Check sheet for the modelled part. Datum: model origin and axes. Units: mm. Face numbers are marked on the shaded views. A direction names the side the tool comes from. Give positions to 0.01 mm unless a question says otherwise; leave off trailing zeros. Order: outer loops, then holes, each group sorted by start corner. A loop starts at its lowest first (then second) coordinate and runs counter-clockwise, first axis right, second up. Notation, with made-up numbers: (-15, 52.5) - (-3, 52.5) arc R21 cw to (-3, 76.5) - close; hole circle Ø4 at (14, -23.75). An arc over 180 degrees is marked (long way). Answer in a Markdown table with one row per item.
from build123d import *

# Parameters (mm, degrees)
SKETCH1_W           = 120
SKETCH1_H           = 86
SKETCH1_W_2         = 10
SKETCH1_H_2         = 60
BOSS_EXTRUDE1_DEPTH = 470


with BuildPart() as part:
    # Sketch1 → Boss-Extrude1 (new body)
    with BuildSketch(Plane(origin=(0, 0, 0), x_dir=(1, 0, 0), z_dir=(0, 1, 0))):
        with BuildLine():
            Line((60, 74.46), (-69.377570777, 74.46))
            ThreePointArc((-69.377570777, 74.46), (-97.633626185, 65.17182404), (-117.46, 43))
            Line((-117.46, 43), (-117.46, -43))
            ThreePointArc((-117.46, -43), (-97.633626185, -65.17182404), (-69.377570777, -74.46))
            Line((-69.377570777, -74.46), (60, -74.46))
            ThreePointArc((60, -74.46), (82.245579336, -65.245579336), (91.46, -43))
            Line((91.46, -43), (91.46, 43))
            ThreePointArc((91.46, 43), (82.245579336, 65.245579336), (60, 74.46))
        make_face()
        Rectangle(SKETCH1_W, SKETCH1_H, mode=Mode.SUBTRACT)
        with Locations((-65.86, 0.020423388)):
            Rectangle(SKETCH1_W_2, SKETCH1_H_2, mode=Mode.SUBTRACT)
        with Locations((-111.1, 0.020423388)):
            Rectangle(SKETCH1_W_2, SKETCH1_H_2, mode=Mode.SUBTRACT)
    extrude(amount=BOSS_EXTRUDE1_DEPTH)


solid = part.part
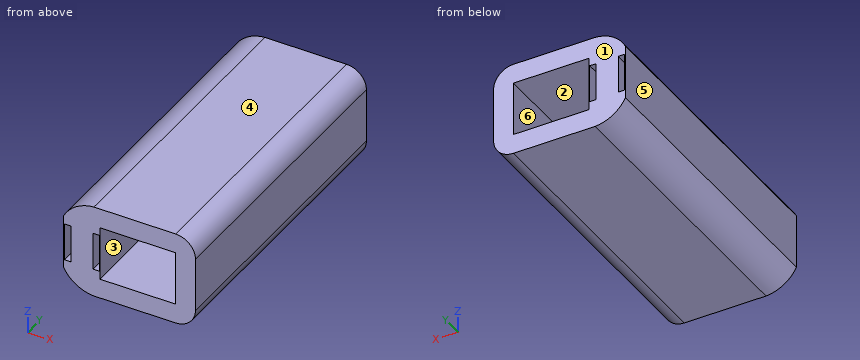
(1) Cross-section at A-A, the plane x = 47.5. Record the cut outline in (y, z).
Geometry says:
| item | result |
|---|---|
| outline | (0, -74.46) - (470, -74.46) - (470, -43) - (0, -43) - close; (0, 43) - (470, 43) - (470, 74.46) - (0, 74.46) - close |
(2) Thickness scan on L1, parallel to X at y = 126.5, z = 0; L2, parallel to Z at x = -39, y = 293.5; L3, parallel to X at y = 207, z = -39. Record the ranges inside material, lowest first.
Geometry says:
| item | result |
|---|---|
| L1 | -117.46 to -116.1, -106.1 to -70.86, -60.86 to -60, 60 to 91.46 |
| L2 | -74.46 to -43, 43 to 74.46 |
| L3 | -117.46 to -60, 60 to 91.46 |
(3) Cross-section at D-D, the plane x = -95.5. Record the cut outline in (y, z).
Geometry says:
| item | result |
|---|---|
| outline | (0, -66.5) - (470, -66.5) - (470, 66.5) - (0, 66.5) - close |
(4) Mould release check, pull along Z, two halves, no side actions. Record for the marked faces 1, 2, 3 and 4: pulls with the +Z half, pulls with the -Z half, needs draft (parallel to the pull), parting line crosses it, or undercut.
Geometry says:
| item | result |
|---|---|
| face 1 | needs draft |
| face 2 | undercut |
| face 3 | undercut |
| face 4 | pulls with the +Z half |
(5) Cross-section at B-B, the plane z = -23. Record the cut outline in (x, y).
Geometry says:
| item | result |
|---|---|
| outline | (-117.46, 0) - (-116.1, 0) - (-116.1, 470) - (-117.46, 470) - close; (-106.1, 0) - (-70.86, 0) - (-70.86, 470) - (-106.1, 470) - close; (-60.86, 0) - (-60, 0) - (-60, 470) - (-60.86, 470) - close; (60, 0) - (91.46, 0) - (91.46, 470) - (60, 470) - close |
(6) Gauge pin test, flat ends, axial feed: P1, Ø5, axis at x = -110, y = 167, coming from the +Z side; P2, Ø11, axis at x = -113.5, y = 191, coming from the -Z side. Record the tip position at first contact, or that the pin passes through.
Geometry says:
| item | result |
|---|---|
| P1 | z = 57.01 |
| P2 | z = -56.49 |
(7) Cross-section at C-C, the plane y = 73. Record the cut outline in (x, z).
Geometry says:
| item | result |
|---|---|
| outline | (-117.46, -43) arc R57.46 ccw to (-69.38, -74.46) - (60, -74.46) arc R31.46 ccw to (91.46, -43) - (91.46, 43) arc R31.46 ccw to (60, 74.46) - (-69.38, 74.46) arc R57.46 ccw to (-117.46, 43) - close; hole (-116.1, -30.02) - (-106.1, -30.02) - (-106.1, 29.98) - (-116.1, 29.98) - close; hole (-70.86, -30.02) - (-60.86, -30.02) - (-60.86, 29.98) - (-70.86, 29.98) - close; hole (-60, -43) - (60, -43) - (60, 43) - (-60, 43) - close |
(8) Access from +Z, -Z, +X, -X, +Y, -Y to the whole of each face (thin tool, end or side, straight path). Record for the marked faces 5 and 6.
Geometry says:
| item | result |
|---|---|
| face 5 | +Z, -Z, -X, +Y, -Y |
| face 6 | +Y, -Y |
